Source: CAD feature listing. Evaluate the final solid. Frame: model axes, mm. A direction names the side the tool comes from. Round coordinates to 2 decimals unless told otherwise and drop trailing zeros. Loops run counter-clockwise (first coordinate to the right, second up) from the corner with the lowest first, then second, coordinate; pieces in that order, holes last.
(1) Mould query, pull axis X, two halves, no side actions, for faces 3 (the flat face through (-15, -15, 5)), 4 (the cylindrical face through (4.84, 32.59, 39.65)), 5 (the flat face through (0, 1, 15)). Classes: pulls with the +X half, pulls with the -X half, needs draft (parallel to the pull), parting line crosses it, or undercut.
(2) Section A-A, the plane z = 5. Return the cut outline in (x, y).
(3) Material intervals for probe 1 along Z at (x, y) = (11, -25.5); probe 2 along Z at (x, y) = (9.5, -34); probe 3 along Y at (x, z) = (8, 7), sorted ascending.
(4) Section B-B, the plane x = 0. Return the cut outline in (y, z), plus the area to 3 significant figures.
(5) Section D-D, the plane z = 36. Return the cut outline in (x, y), plus the area to 3 significant figures.
(6) Set-up query: faces 1 (the cylindrical face through (0, -40, 7)), 2 (the flat face through (0, -15, 10)). Return all of +Z, -Z, +X, -X, +Y, -Y with unobstructed straight access to the full face (end or side cutting, diameter ignored); none if empty.
(7) Section C-C, the plane y = -17.5. Return the cut outline in (x, z), plus the area to 3 significant figures.
(8) First-contact query: pin 1 Ø12 at (x, z) = (0.5, 35.5) entering from +Y; pin 2 Ø2 at (x, z) = (5.5, 22) entering from -Y; pin 3 Ø11 at (x, z) = (7.5, 4.5) entering from +Y; pin 4 Ø12 at (y, z) = (9, 28) entering from +X. Flat tips, straight axial feed; report the tip coordinate or a pass-through.
```python
from build123d import *

# Parameters (mm, degrees)
CROQUIS1_R              = 40
SALIENTE_EXTRUIR1_DEPTH = 15
CROQUIS3_R              = 9
SALIENTE_EXTRUIR2_DEPTH = 50
CROQUIS4_W              = 30
CROQUIS4_H              = 30
CORTAR_EXTRUIR1_DEPTH   = 10
CORTAR_EXTRUIR3_DEPTH   = 76.498344353


with BuildPart() as part:
    # Croquis1 → Saliente-Extruir1 (new body)
    with BuildSketch(Plane.XY):
        Circle(CROQUIS1_R)
    extrude(amount=SALIENTE_EXTRUIR1_DEPTH)

    # Croquis3 → Saliente-Extruir2 (add)
    with BuildSketch(Plane.XY.offset(15)):
        with Locations((0, 25)):
            Circle(CROQUIS3_R)
    extrude(amount=SALIENTE_EXTRUIR2_DEPTH)

    # Croquis4 → Cortar-Extruir1 (cut)
    with BuildSketch(Plane(origin=(0, 0, 0), x_dir=(-1, 0, 0), z_dir=(0, 0, -1))):
        with Locations((0, -15)):
            Rectangle(CROQUIS4_W, CROQUIS4_H)
    extrude(amount=-CORTAR_EXTRUIR1_DEPTH, mode=Mode.SUBTRACT)

    # Croquis5 → Cortar-Extruir3 (cut, through all)
    with BuildSketch(Plane.XY.offset(15)):
        with BuildLine():
            Line((-17, 36.20773398), (-17, -36.20773398))
            ThreePointArc((-17, -36.20773398), (-40, 0), (-17, 36.20773398))
        make_face()
        with BuildLine():
            Line((17, 36.20773398), (17, -36.20773398))
            ThreePointArc((17, -36.20773398), (40, 0), (17, 36.20773398))
        make_face()
    extrude(amount=-CORTAR_EXTRUIR3_DEPTH, mode=Mode.SUBTRACT)


solid = part.part
```
Output values:
1. face 3: undercut
1. face 4: parting line crosses it
1. face 5: needs draft
2. outline: (-17, -36.21) arc R40 ccw to (17, -36.21) - (17, 36.21) arc R40 ccw to (-17, 36.21) - close; hole (-15, -30) - (15, -30) - (15, 0) - (-15, 0) - close
3. probe 1: z = 10 to 15
3. probe 2: z = 0 to 15
3. probe 3: y = -39.19 to -30, 0 to 39.19
4. outline: (-40, 0) - (-30, 0) - (-30, 10) - (0, 10) - (0, 0) - (40, 0) - (40, 15) - (34, 15) - (34, 65) - (16, 65) - (16, 15) - (-40, 15) - close
4. area: 1,800 mm2
5. outline: circle Ø18 at (0, 25)
5. area: 254 mm2
6. face 1: +Z, -Z, -Y
6. face 2: -Z
7. outline: (-17, 0) - (-15, 0) - (-15, 10) - (15, 10) - (15, 0) - (17, 0) - (17, 15) - (-17, 15) - close
7. area: 210 mm2
8. pin 1: stops at y = 34
8. pin 2: stops at y = 17.21
8. pin 3: stops at y = 39.95
8. pin 4: passes through
